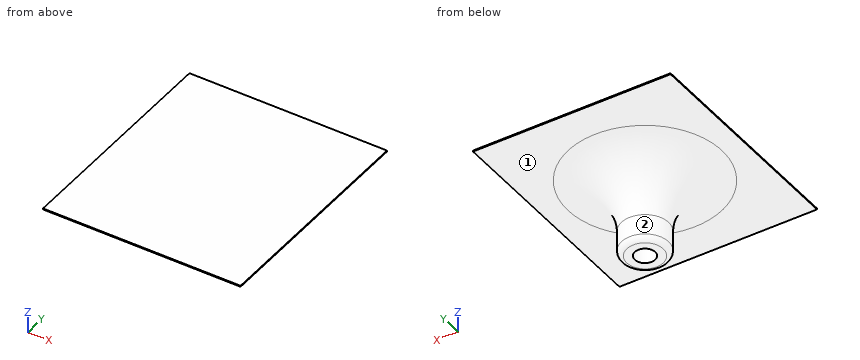
```python
from build123d import *

# Parameters (mm, degrees)
BOSS_EXTRUDE1_START       = -19.05
BOSS_EXTRUDE1_OUTLINE_R   = 5.588
BOSS_EXTRUDE1_OUTLINE_R_2 = 2.413
BOSS_EXTRUDE1_DEPTH       = 19.05
SKETCH16_W                = 47
SKETCH16_H                = 53.5
BOSS_EXTRUDE2_DEPTH       = 0.254
FILLET1_R                 = 12.7
FILLET3_R                 = 1.27


# Read off the part's stored shape, not the designer's step: Boss-Extrude1
with BuildPart() as part:
    # Boss-Extrude1 outline → Boss-Extrude1 (new body)
    with BuildSketch(Plane.XY.offset(BOSS_EXTRUDE1_START)):
        Circle(BOSS_EXTRUDE1_OUTLINE_R)
        Circle(BOSS_EXTRUDE1_OUTLINE_R_2, mode=Mode.SUBTRACT)
    extrude(amount=BOSS_EXTRUDE1_DEPTH)

    # Sketch16 → Boss-Extrude2 (add)
    with BuildSketch(Plane.XY):
        Rectangle(SKETCH16_W, SKETCH16_H)
    extrude(amount=-BOSS_EXTRUDE2_DEPTH)

    # Fillet1
    fillet1_edges = [part.edges().sort_by_distance(p)[0] for p in [
        (-5.588, 0, -0.254),
    ]]
    fillet(fillet1_edges, radius=FILLET1_R)

    # Fillet3
    fillet3_edges = [part.edges().sort_by_distance(p)[0] for p in [
        (-5.588, 0, -19.05),
    ]]
    fillet(fillet3_edges, radius=FILLET3_R)


solid = part.part
```
CAD build for the part. Positions are in the model's coordinates, mm. Face numbers are marked on the shaded views. Coordinates: 2 decimals unless noted, no trailing zeros. Order: outer loops, then holes, each group sorted by start corner. A loop starts at its lowest first (then second) coordinate and runs counter-clockwise, first axis right, second up. Notation, with made-up numbers: (13, 21) - (22, 21) arc R13 ccw to (22, 44) - close; hole circle Ø1 at (51.5, -9). An arc over 180 degrees is marked (long way). Use a Markdown table: item, result. Add a question column.
(1) Saw through at A-A (y = 0). Give the cut face in (x, z), then the cut area to 3 significant figures.
(2) Flat gauge pins, fed straight in: pin 1 (3 mm diameter, centred on x = 17.5, y = -5, fed in from +Z); pin 2 (1.4 mm diameter, centred on x = -1, y = 1, fed in from -Z); pin 3 (8 mm diameter, centred on x = 5.5, z = -6, fed in from -Y); pin 4 (1 mm diameter, centred on y = -8, z = -11, fed in from -X). Where does each tip first touch, or does it go through?
(3) Saw through at D-D (y = -23). Give the cut face in (x, z), then the cut area to 3 significant figures.
(4) Saw through at B-B (x = 0). Give the cut face in (y, z), then the cut area to 3 significant figures.
(5) Pull direction Y, two halves, no side cores. Call the marked faces 1 and 2: +Y half, -Y half, draft (parallel to the pull), parting line (faces both ways), or undercut.
(6) Drill centre lines: line 1 along X through (y, z) = (0, -14.5); line 2 along Z through (x, y) = (14, -18). Where is each one in solid material? Low to high. Write a range as [from, to].
(7) Saw through at C-C (z = -14.75). Give the cut face in (x, y).
Solved:
| question | item | result |
|---|---|---|
| 1 | outline | (-23.5, -0.25) - (-18.29, -0.25) arc R12.7 cw to (-5.59, -12.95) - (-5.59, -17.78) arc R1.27 ccw to (-4.32, -19.05) - (-2.41, -19.05) - (-2.41, -0.25) - (2.41, -0.25) - (2.41, -19.05) - (4.32, -19.05) arc R1.27 ccw to (5.59, -17.78) - (5.59, -12.95) arc R12.7 cw to (18.29, -0.25) - (23.5, -0.25) - (23.5, 0) - (-23.5, 0) - close |
| 1 | area | 200 mm² |
| 2 | pin 1 | stops at z = 0 |
| 2 | pin 2 | stops at z = -0.25 |
| 2 | pin 3 | stops at y = -10.75 |
| 2 | pin 4 | passes through |
| 3 | outline | (-23.5, -0.25) - (23.5, -0.25) - (23.5, 0) - (-23.5, 0) - close |
| 3 | area | 11.9 mm² |
| 4 | outline | (-26.75, -0.25) - (-18.29, -0.25) arc R12.7 cw to (-5.59, -12.95) - (-5.59, -17.78) arc R1.27 ccw to (-4.32, -19.05) - (-2.41, -19.05) - (-2.41, -0.25) - (2.41, -0.25) - (2.41, -19.05) - (4.32, -19.05) arc R1.27 ccw to (5.59, -17.78) - (5.59, -12.95) arc R12.7 cw to (18.29, -0.25) - (26.75, -0.25) - (26.75, 0) - (-26.75, 0) - close |
| 4 | area | 201 mm² |
| 5 | face 1 | draft |
| 5 | face 2 | parting line |
| 6 | line 1 | x = [-5.59, -2.41], [2.41, 5.59] |
| 6 | line 2 | z = [-0.25, 0] |
| 7 | outline | circle Ø11.18 at (0, 0); hole circle Ø4.83 at (0, 0) |
